Print and shaded views of the part. All mm, measured from the part's lowest x, y and z. Round coordinates to 2 decimals unless told otherwise and drop trailing zeros. Loops run counter-clockwise (first coordinate to the right, second up) from the corner with the lowest first, then second, coordinate; pieces in that order, holes last. Notation, with made-up numbers: (74, -7.5) -> (94, -7.5) arc R13 ccw to (94, 8.5) -> close; hole circle Ø5 at (33, 27.5). An arc over 180 degrees is marked (long way). Use a Markdown table: item, result.
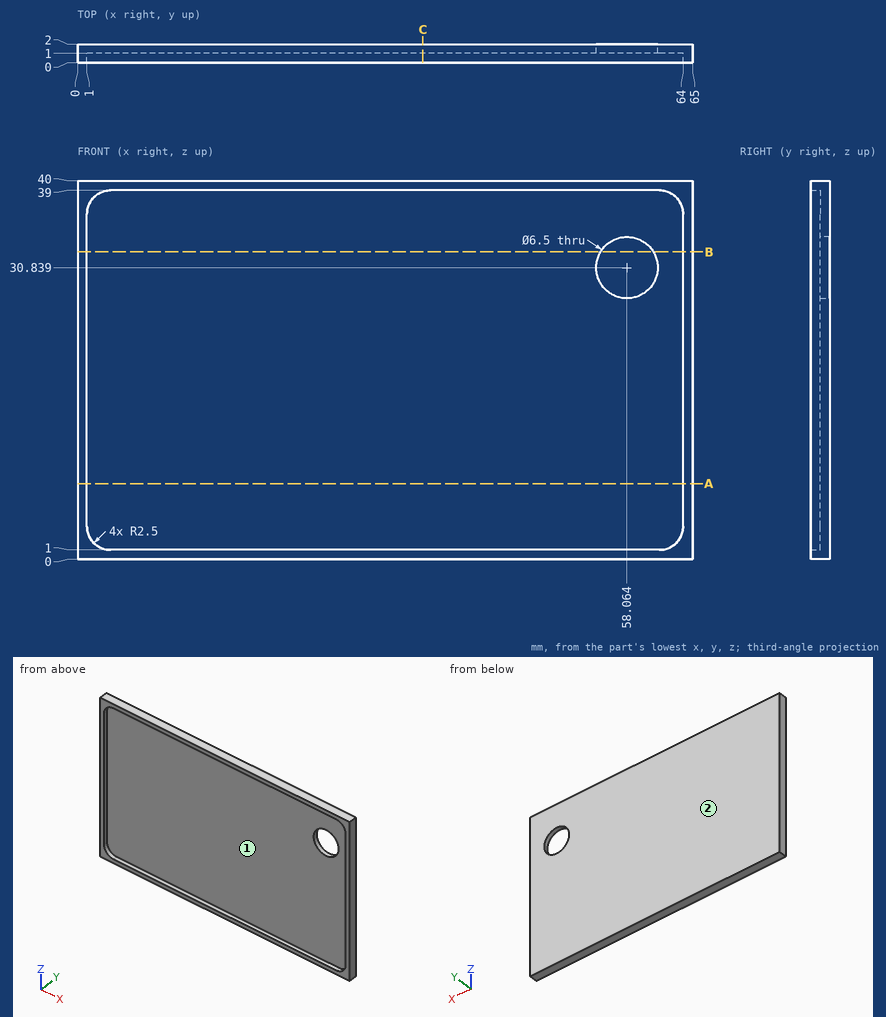
Q1. Band-saw the part on C-C, the plane x = 36.5. Give the cut face in (y, z).
Results list:
| item | result |
|---|---|
| outline | (0, 0) -> (2, 0) -> (2, 40) -> (0, 40) -> (0, 39) -> (1, 39) -> (1, 1) -> (0, 1) -> close |
Q2. Pull direction Z, two halves, no side cores. Call the marked faces 1 and 2: released by +Z, released by -Z, zero draft, split by the parting line, or undercut.
Results list:
| item | result |
|---|---|
| face 1 | undercut |
| face 2 | zero draft |
Q3. Flat gauge pin, fed straight in: pin 1 (8 mm diameter, centred on x = 24, z = 23, fed in from -Y). Where does the tip first touch, or does it go through?
Results list:
| item | result |
|---|---|
| pin 1 | stops at y = 1 |
Q4. Band-saw the part on B-B, the plane z = 32.5. Give the cut face in (x, y).
Results list:
| item | result |
|---|---|
| outline | (0, 0) -> (1, 0) -> (1, 1) -> (55.27, 1) -> (55.27, 2) -> (0, 2) -> close; (60.86, 1) -> (64, 1) -> (64, 0) -> (65, 0) -> (65, 2) -> (60.86, 2) -> close |
Q5. Drill centre lines: L1, parallel to Z at x = 23, y = 0.4; L2, parallel to X at y = 0.9, z = 19; L3, parallel to Y at x = 6, z = 23. Where is each one in solid material? Low to high. Write a range as from..to.
Results list:
| item | result |
|---|---|
| L1 | z = 0..1, 39..40 |
| L2 | x = 0..1, 64..65 |
| L3 | y = 1..2 |
Q6. Band-saw the part on A-A, the plane z = 8. Give the cut face in (x, y).
Results list:
| item | result |
|---|---|
| outline | (0, 0) -> (1, 0) -> (1, 1) -> (64, 1) -> (64, 0) -> (65, 0) -> (65, 2) -> (0, 2) -> close |
